from build123d import *

# Parameters (mm, degrees)
BOSS_EXTRUDE1_DEPTH     = 15
SCALE4_SCALE            = 10
SHELL3_T                = -1
SKETCH7_R               = 2.5
CUT_EXTRUDE2_DEPTH      = 1
CUT_EXTRUDE2_DEPTH_BACK = 151
SKETCH8_R               = 2.5
CUT_EXTRUDE3_DEPTH      = 1
CUT_EXTRUDE3_DEPTH_BACK = 151
SKETCH11_R              = 6
CUT_EXTRUDE5_DEPTH      = 1
CUT_EXTRUDE5_DEPTH_BACK = 151
SKETCH12_R              = 6
CUT_EXTRUDE6_DEPTH      = 1
CUT_EXTRUDE6_DEPTH_BACK = 151
SKETCH19_W              = 20
SKETCH19_H              = 148
BOSS_EXTRUDE6_DEPTH     = 12
SKETCH6_R               = 3.1
CUT_EXTRUDE9_DEPTH      = 1
CUT_EXTRUDE9_DEPTH_BACK = 151
SKETCH22_R              = 7.95
CUT_EXTRUDE10_DEPTH     = 2


with BuildPart() as part:
    # Sketch1 → Boss-Extrude1 (new body)
    with BuildSketch(Plane.XY):
        Polygon((-49.791399094, 32.645333647), (-19.791399094, 32.645333647), (-19.791399094, 29.645333647), (-22.238991949, 22.388566018), (-47.247714564, 22.388566018), (-49.791399094, 29.645333647), align=None)
    extrude(amount=BOSS_EXTRUDE1_DEPTH)


with BuildPart() as part_1:
    # Scale4: scaled about (-34.775342822, 27.686391484, 7.5)
    add(part.part.scale(SCALE4_SCALE).moved(Location((312.978085398, -249.177523356, -67.5))))

    # Shell3
    shell3_openings = [part_1.faces().sort_by_distance(p)[0] for p in [
        (-34.935905541, 77.275813113, 7.5),
    ]]
    offset(amount=SHELL3_T, openings=shell3_openings, kind=Kind.INTERSECTION)

    # Sketch7 → Cut-Extrude2 (cut, two sides)
    with BuildSketch(Plane.XY.offset(82.5)) as cut_extrude2_sk:
        with Locations((40.588165903, -17.79186318)):
            Circle(SKETCH7_R)
    extrude(amount=CUT_EXTRUDE2_DEPTH, mode=Mode.SUBTRACT)
    extrude(cut_extrude2_sk.sketch, amount=-CUT_EXTRUDE2_DEPTH_BACK, mode=Mode.SUBTRACT)

    # Sketch8 → Cut-Extrude3 (cut, two sides)
    with BuildSketch(Plane.XY.offset(82.5)) as cut_extrude3_sk:
        with Locations((-34.935905541, 27.275813113)):
            Circle(SKETCH8_R)
    extrude(amount=CUT_EXTRUDE3_DEPTH, mode=Mode.SUBTRACT)
    extrude(cut_extrude3_sk.sketch, amount=-CUT_EXTRUDE3_DEPTH_BACK, mode=Mode.SUBTRACT)

    # Sketch11 → Cut-Extrude5 (cut, two sides)
    with BuildSketch(Plane(origin=(0, 0, -67.5), x_dir=(-1, 0, 0), z_dir=(0, 0, -1))) as cut_extrude5_sk:
        with Locations((-40.588165903, -17.79186318)):
            Circle(SKETCH11_R)
    extrude(amount=CUT_EXTRUDE5_DEPTH, mode=Mode.SUBTRACT)
    extrude(cut_extrude5_sk.sketch, amount=-CUT_EXTRUDE5_DEPTH_BACK, mode=Mode.SUBTRACT)

    # Sketch12 → Cut-Extrude6 (cut, two sides)
    with BuildSketch(Plane.XY.offset(82.5)) as cut_extrude6_sk:
        with Locations((-34.935905541, 27.275813113)):
            Circle(SKETCH12_R)
    extrude(amount=CUT_EXTRUDE6_DEPTH, mode=Mode.SUBTRACT)
    extrude(cut_extrude6_sk.sketch, amount=-CUT_EXTRUDE6_DEPTH_BACK, mode=Mode.SUBTRACT)

    # Sketch19 → Boss-Extrude6 (add)
    with BuildSketch(Plane(origin=(0, -24.29186318, 0), x_dir=(1, 0, 0), z_dir=(0, 1, 0))):
        with Locations((-109.499060243, -7.5)):
            Rectangle(SKETCH19_W, SKETCH19_H)
    extrude(amount=BOSS_EXTRUDE6_DEPTH)

    # Sketch6 → Cut-Extrude9 (cut, two sides)
    with BuildSketch(Plane.XY.offset(82.5)) as cut_extrude9_sk:
        with Locations((-109.499060243, -17.79186318)):
            Circle(SKETCH6_R)
    extrude(amount=CUT_EXTRUDE9_DEPTH, mode=Mode.SUBTRACT)
    extrude(cut_extrude9_sk.sketch, amount=-CUT_EXTRUDE9_DEPTH_BACK, mode=Mode.SUBTRACT)

    # Sketch22 → Cut-Extrude10 (cut)
    with BuildSketch(Plane(origin=(115.064094459, 0, 0), x_dir=(0, 0, -1), z_dir=(1, 0, 0))):
        with Locations((-20.75, 62.275813113)):
            Circle(SKETCH22_R)
        with Locations((5.75, 62.275813113)):
            Circle(SKETCH22_R)
    extrude(amount=-CUT_EXTRUDE10_DEPTH, mode=Mode.SUBTRACT)


solid = part_1.part
Read the model definition and answer for the solid it produces. Units are mm, in the model's axes. A direction names the side the tool comes from. Round coordinates to 2 decimals unless told otherwise and drop trailing zeros. Loops run counter-clockwise (first coordinate to the right, second up) from the corner with the lowest first, then second, coordinate; pieces in that order, holes last.
Q1. Section B-B on x = -51 is taken. Write down the section's boundary in (y, z).
Q2. Determine the mould class of faces 1 (the face through (-139, -24.292, 6)), 2 (the face through (-35.717, 33.225, 82.007)), 3 (the face through (114.064, 63, 6)) for opening direction Y: released by +Y, released by -Y, zero draft, split by the parting line, or undercut.
Q3. Section A-A on z = 20.75 is taken. Write down the section's boundary in (x, y), and give its area (3 significant figures).
Q4. Each of these flat-tipped pins is pushed along its axis until it touches: pin 1 (6 mm diameter, centred on y = -18, z = 35.5, fed in from +X); pin 2 (9.5 mm diameter, centred on y = -16, z = 19.5, fed in from -X); pin 3 (19.5 mm diameter, centred on x = -138.5, z = 1, fed in from +Y). Where does it stop, or does it pass through?
Q5. Section D-D on y = 16 is taken. Write down the section's boundary in (x, z).
Q6. Section C-C on z = -43.5 is taken. Write down the section's boundary in (x, y), and give its area (3 significant figures).
Q7. Consider probe 1 along X at (y, z) = (56, -55); probe 2 along Z at (x, y) = (-133, 43); probe 3 along Y at (x, z) = (-94, 41). Determine where each line is inside the solid, lowest interval first.
Q8. Which of the six approach directions +Z, -Z, +X, -X, +Y, -Y give full straight-line access (tool end or side, diameter ignored) to faces 4 (the face through (-119.499, -18, 9)), 5 (the face through (114.571, 54.515, -4.027)), 6 (the face through (-33, 38, -67.5))?
Output:
1. outline: (-25.29, -67.5) - (77.28, -67.5) - (77.28, -66.5) - (-24.29, -66.5) - (-24.29, 81.5) - (77.28, 81.5) - (77.28, 82.5) - (-25.29, 82.5) - close
2. face 1: released by +Y
2. face 2: undercut
2. face 3: zero draft
3. outline: (-184.94, 47.28) - (-159.5, -25.29) - (90.59, -25.29) - (115.06, 47.28) - (115.06, 54.33) - (114.06, 54.33) - (114.06, 47.44) - (89.87, -24.29) - (-99.5, -24.29) - (-99.5, -12.29) - (-119.5, -12.29) - (-119.5, -24.29) - (-158.79, -24.29) - (-183.94, 47.45) - (-183.94, 77.28) - (-184.94, 77.28) - close; (114.06, 70.23) - (115.06, 70.23) - (115.06, 77.28) - (114.06, 77.28) - close; hole circle Ø6.2 at (-109.5, -17.79)
3. area: 656 mm2
4. pin 1: stops at x = 94.06
4. pin 2: stops at x = -164.42
4. pin 3: stops at y = -24.29
5. outline: (-173.97, -67.5) - (104.52, -67.5) - (104.52, 82.5) - (-173.97, 82.5) - close; hole (-172.91, -66.5) - (103.46, -66.5) - (103.46, 81.5) - (-172.91, 81.5) - close
6. outline: (-184.94, 47.28) - (-159.5, -25.29) - (90.59, -25.29) - (115.06, 47.28) - (115.06, 77.28) - (114.06, 77.28) - (114.06, 47.44) - (89.87, -24.29) - (-99.5, -24.29) - (-99.5, -12.29) - (-119.5, -12.29) - (-119.5, -24.29) - (-158.79, -24.29) - (-183.94, 47.45) - (-183.94, 77.28) - (-184.94, 77.28) - close; hole circle Ø6.2 at (-109.5, -17.79)
6. area: 672 mm2
7. probe 1: x = -184.94 to -183.94, 114.06 to 115.06
7. probe 2: z = -67.5 to -66.5, 81.5 to 82.5
7. probe 3: y = -25.29 to -24.29
8. face 4: +Y
8. face 5: +X
8. face 6: -Z, +X, -X, +Y, -Y
